from build123d import *

# Parameters (mm, degrees)
SKETCH1_R           = 3.5
SKETCH1_R_2         = 1.5
SKETCH1_R_3         = 10
BOSS_EXTRUDE1_DEPTH = 4
SKETCH2_R           = 6
BOSS_EXTRUDE2_DEPTH = 12.3
SKETCH3_R           = 7.5
BOSS_EXTRUDE3_DEPTH = 0.5
SKETCH4_W           = 3
SKETCH4_H           = 8
BOSS_EXTRUDE4_DEPTH = 24.2
SKETCH5_R           = 5
BOSS_EXTRUDE5_DEPTH = 10


with BuildPart() as part:
    # Sketch1 → Boss-Extrude1 (new body)
    # profile 1 of 7: a face of its own
    with BuildSketch(Plane.XY):
        with Locations((0, -13.5)):
            Circle(SKETCH1_R)
        with Locations((0, -13.5)):
            Circle(SKETCH1_R_2, mode=Mode.SUBTRACT)
    # profile 2 of 7: a face of its own
    with BuildSketch(Plane.XY):
        with BuildLine():
            ThreePointArc((8.764562642, -4.814814815), (5.091750776, -8.606629656), (9e-09, -10))
            ThreePointArc((9e-09, -10), (2.474873737, -11.025126269), (3.5, -13.5))
            ThreePointArc((3.5, -13.5), (3.390176193, -14.369888143), (3.067596925, -15.185185185))
            Line((3.067596925, -15.185185185), (8.764562642, -4.814814815))
        make_face()
    # profile 3 of 7: a face of its own
    with BuildSketch(Plane.XY):
        Circle(SKETCH1_R_3)
    # profile 4 of 7: a face of its own
    with BuildSketch(Plane.XY):
        with BuildLine():
            Line((8.764562642, 4.814814815), (3.067596925, 15.185185185))
            ThreePointArc((3.067596925, 15.185185185), (3.390176193, 14.369888143), (3.5, 13.5))
            ThreePointArc((3.5, 13.5), (2.474873734, 11.025126266), (0, 10))
            ThreePointArc((0, 10), (5.091750772, 8.606629658), (8.764562642, 4.814814815))
        make_face()
    # profile 5 of 7: a face of its own
    with BuildSketch(Plane.XY):
        with Locations((0, 13.5)):
            Circle(SKETCH1_R)
        with Locations((0, 13.5)):
            Circle(SKETCH1_R_2, mode=Mode.SUBTRACT)
    # profile 6 of 7: a face of its own
    with BuildSketch(Plane.XY):
        with BuildLine():
            ThreePointArc((0, 10), (-3.01232038, 11.71788723), (-3.067596925, 15.185185185))
            Line((-3.067596925, 15.185185185), (-8.764562642, 4.814814815))
            ThreePointArc((-8.764562642, 4.814814815), (-5.091750772, 8.606629658), (0, 10))
        make_face()
    # profile 7 of 7: a face of its own
    with BuildSketch(Plane.XY):
        with BuildLine():
            ThreePointArc((9e-09, -10), (-5.091750768, -8.606629661), (-8.764562642, -4.814814815))
            Line((-8.764562642, -4.814814815), (-3.067596925, -15.185185185))
            ThreePointArc((-3.067596925, -15.185185185), (-3.012320378, -11.717887226), (9e-09, -10))
        make_face()
    extrude(amount=BOSS_EXTRUDE1_DEPTH)

    # Sketch2 → Boss-Extrude2 (add)
    with BuildSketch(Plane.XY.offset(4)):
        Circle(SKETCH2_R)
    extrude(amount=BOSS_EXTRUDE2_DEPTH)

    # Sketch3 → Boss-Extrude3 (add)
    with BuildSketch(Plane(origin=(0, 0, 0), x_dir=(-1, 0, 0), z_dir=(0, 0, -1))):
        with Locations(Location((0, 0, 0), (0, 0, 180))):
            Circle(SKETCH3_R)
    extrude(amount=BOSS_EXTRUDE3_DEPTH)

    # Sketch4 → Boss-Extrude4 (add)
    with BuildSketch(Plane(origin=(0, 0, -0.5), x_dir=(-1, 0, 0), z_dir=(0, 0, -1))):
        Rectangle(SKETCH4_W, SKETCH4_H)
    extrude(amount=BOSS_EXTRUDE4_DEPTH)

    # Sketch5 → Boss-Extrude5 (add)
    with BuildSketch(Plane(origin=(0, 0, -0.5), x_dir=(-1, 0, 0), z_dir=(0, 0, -1))):
        Circle(SKETCH5_R)
    extrude(amount=BOSS_EXTRUDE5_DEPTH)


solid = part.part
The model under review builds one solid part; all positions refer to its coordinate system, in mm. A direction names the side the tool comes from. Round coordinates to 2 decimals unless told otherwise and drop trailing zeros. Write each loop counter-clockwise with the first axis right and the second up, starting at its lowest first coordinate (ties: lowest second). Pieces come first, ordered by that corner, then holes. Notation, with made-up numbers: M 10.25,55 L 51.25,55 A16 ccw 51.25,65 Z; hole C 44.25,60 d9. An arc over 180 degrees is marked long. Answer as CSV lines item,"result". Start each with the question number.
Q1. Consider section C-C, the plane y = 0. Give the boundary of the cut face in (x, z).
Q2. Consider section D-D, the plane y = 13.5. Give the boundary of the cut face in (x, z), then the cut area to 3 significant figures.
Q3. Consider section B-B, the plane z = 1. Give the boundary of the cut face in (x, y).
Q4. Wall thickness on line 1 along Z through (x, y) = (-2, 2.5); line 2 along Z through (x, y) = (3, 9); line 3 along Y through (x, z) = (4.75, 3.5): over which ranges is each line inside the solid? List them lowest first.
Q5. Consider section A-A, the plane x = 0. Give the boundary of the cut face in (y, z), then the cut area to 3 significant figures.
Q6. Clearance check with flat-ended pins moving along their axes: P1, Ø1.5, axis at x = -0.5, z = -20.5, coming from the -Y side; P2, Ø2, axis at x = 5.5, z = -10, coming from the -Y side; P3, Ø8, axis at y = -11.5, z = -14.5, coming from the +X side; P4, Ø2.5, axis at y = 0.5, z = -20.5, coming from the -X side. State where each tip first meets the part, or that it passes through.
Q7. The part is to be moulded in two halves that separate along X. For faces 4 (the face through (2, 5, -0.5)), 5 (the face through (-10, 0, 2)), 6 (the face through (0, -15, 2)), say which applies: +X half, -X half, draft (parallel to the pull), parting line (faces both ways), or undercut.
Q8. Tool access review of faces 1 (the face through (1.5, 0, -18)), 2 (the face through (-1.5, 0, -18)), 3 (the face through (0, 8, 0)): name each direction out of +Z, -Z, +X, -X, +Y, -Y from which nothing blocks a thin tool from reaching the whole face with its end or side.
Result set:
1,outline,"M -10,0 L -7.5,0 L -7.5,-0.5 L -5,-0.5 L -5,-10.5 L -1.5,-10.5 L -1.5,-24.7 L 1.5,-24.7 L 1.5,-10.5 L 5,-10.5 L 5,-0.5 L 7.5,-0.5 L 7.5,0 L 10,0 L 10,4 L 6,4 L 6,16.3 L -6,16.3 L -6,4 L -10,4 Z"
2,outline,"M -3.99,0 L -1.5,0 L -1.5,4 L -3.99,4 Z; M 1.5,0 L 3.99,0 L 3.99,4 L 1.5,4 Z"
2,area,"19.9 mm²"
3,outline,"M -8.76,-4.81 L -3.07,-15.19 A3.5 ccw 3.07,-15.19 L 8.76,-4.81 A10 ccw 8.76,4.81 L 3.07,15.19 A3.5 ccw -3.07,15.19 L -8.76,4.81 A10 ccw Z; hole C 0,-13.5 d3; hole C 0,13.5 d3"
4,line 1,"z = -10.5 to 16.3"
4,line 2,"z = 0 to 4"
4,line 3,"y = -12.12 to 12.12"
5,outline,"M -17,0 L -15,0 L -15,4 L -17,4 Z; M -12,0 L -7.5,0 L -7.5,-0.5 L -5,-0.5 L -5,-10.5 L -4,-10.5 L -4,-24.7 L 4,-24.7 L 4,-10.5 L 5,-10.5 L 5,-0.5 L 7.5,-0.5 L 7.5,0 L 12,0 L 12,4 L 6,4 L 6,16.3 L -6,16.3 L -6,4 L -12,4 Z; M 15,0 L 17,0 L 17,4 L 15,4 Z"
5,area,"481 mm²"
6,P1,"stops at y = -4"
6,P2,"stops at y = -2.18"
6,P3,"passes through"
6,P4,"stops at x = -1.5"
7,face 4,"draft"
7,face 5,"-X half"
7,face 6,"undercut"
8,face 1,"-Z, +X, +Y, -Y"
8,face 2,"-Z, -X, +Y, -Y"
8,face 3,"-Z"
